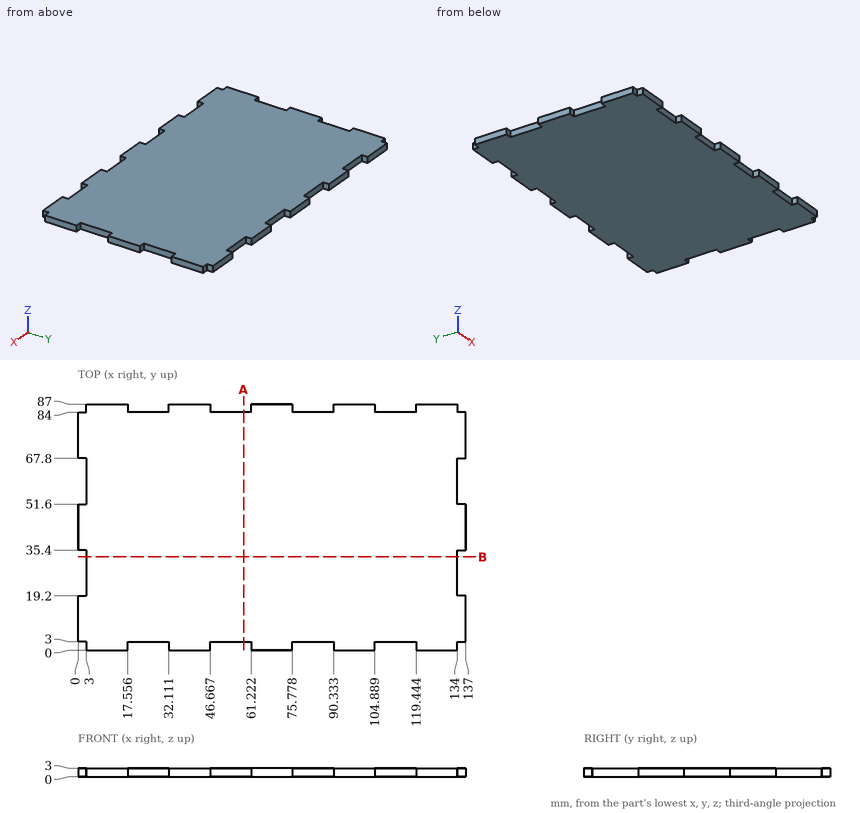
Check sheet for the drawn part. Datum: minimum x, y, z corner. Units: mm. Round coordinates to 2 decimals unless told otherwise and drop trailing zeros. Write each loop counter-clockwise with the first axis right and the second up, starting at its lowest first coordinate (ties: lowest second). Pieces come first, ordered by that corner, then holes. Notation, with made-up numbers: (89.25, 85) -> (141.25, 85) arc R8 cw to (141.25, 94) -> close; hole circle Ø11 at (31.5, -25). An arc over 180 degrees is marked (long way). Put each result on its own line as item: value.
(1) Sectioned sample at A-A (x = 58.5). Enter the section's corners in (y, z).
Values found:
outline: (3, 0) -> (84, 0) -> (84, 3) -> (3, 3) -> close
(2) Go/stop test with flat-tipped pins: pin 1 Ø1.5 at (y, z) = (2, 2) entering from -X; pin 2 Ø1.5 at (y, z) = (2, 2) entering from +X; pin 3 Ø1.5 at (x, z) = (1, 1.5) entering from +Y. Record where each tip stops, or that it passes through.
Values found:
pin 1: stops at x = 3
pin 2: stops at x = 134
pin 3: stops at y = 84
(3) Sectioned sample at B-B (y = 33). Enter the section's corners in (x, z), plus the area to 3 significant figures.
Values found:
outline: (3, 0) -> (134, 0) -> (134, 3) -> (3, 3) -> close
area: 393 mm^2
(4) Material ranges on line 1 (X direction, y = 28.5, z = 2.6); line 2 (Y direction, x = 57, z = 0.2), recorded low to high.
Values found:
line 1: x = 3 to 134
line 2: y = 3 to 84
